Part model, mm, in its own coordinate system. A direction names the side the tool comes from. Give positions to 0.01 mm unless a question says otherwise; leave off trailing zeros. Loops run counter-clockwise (first coordinate to the right, second up) from the corner with the lowest first, then second, coordinate; pieces in that order, holes last. Notation, with made-up numbers: (20, 14.25) -> (28, 14.25) arc R8 ccw to (28, 24.25) -> close; hole circle Ø3 at (12, 44.5). An arc over 180 degrees is marked (long way). Write item = value, one per line.
from build123d import *

# Parameters (mm, degrees)
F1_R      = 47.625
F2_DEPTH  = 25.4
F0_R      = 88.9
F2_FACE_R = 47.625
F3_DEPTH  = 6.35
F4_R      = 5.08
F5_SIZE   = 2.54
F6_R      = 82.55
F6_R_2    = 57.15
F8_DEPTH  = 3.175
F7_R      = 41.275
F9_DEPTH  = 25.4
F10_R     = 1.524


with BuildPart() as f2:
    # F1 (on Top) → F2 (new body)
    with BuildSketch(Plane.XY):
        Circle(F1_R)
    extrude(amount=F2_DEPTH)

    # F0 (on Top) + F2_face (on face) → F3 (join)
    with BuildSketch(Plane.XY):
        Circle(F0_R)
    with BuildSketch(Plane.XY.offset(25.4)):
        Circle(F2_FACE_R)
    extrude(amount=-F3_DEPTH)

    # F4
    f4_edges = [f2.edges().sort_by_distance(p)[0] for p in [
        (-88.9, 0, -6.35),
    ]]
    fillet(f4_edges, radius=F4_R)

    # F5
    f5_edges = [f2.edges().sort_by_distance(p)[0] for p in [
        (-47.625, 0, 25.4),
    ]]
    chamfer(f5_edges, length=F5_SIZE)

    # F6 (on Top) → F8 (cut)
    with BuildSketch(Plane.XY):
        Circle(F6_R)
        Circle(F6_R_2, mode=Mode.SUBTRACT)
    extrude(amount=-F8_DEPTH, mode=Mode.SUBTRACT)

    # F7 (on Top) → F9 (cut)
    with BuildSketch(Plane.XY):
        Circle(F7_R)
    extrude(amount=F9_DEPTH, mode=Mode.SUBTRACT)

    # F10
    f10_edges = [f2.edges().sort_by_distance(p)[0] for p in [
        (-82.55, 0, -3.175),
        (-57.15, 0, -3.175),
        (-47.625, 0, 0),
    ]]
    fillet(f10_edges, radius=F10_R)


solid = f2.part
1) Drill centre lines: line 1 along Y through (x, z) = (0, -1); line 2 along Y through (x, z) = (0, 9) (3 decimals); line 3 along X through (y, z) = (-32.5, -1). Where is each one in solid material? Low to high. Write a range as [from, to].
Resolved:
line_1 = [-88.9, -82.55], [-57.15, 57.15], [82.55, 88.9]
line_2 = [-47.625, -41.275], [41.275, 47.625]
line_3 = [-82.75, -75.88], [-47.01, 47.01], [75.88, 82.75]
2) Pull direction X, two halves, no side cores. Call faces 3 (the face through (-1, 1, 0)), 4 (the face through (20, -37, 25.4)), 5 (the face through (-37.794, -28.979, 12.043)), 6 (the face through (-17.895, -80.587, -0.814)): pulls with the +X half, pulls with the -X half, needs draft (parallel to the pull), parting line crosses it, or undercut.
Resolved:
face_3 = undercut
face_4 = needs draft
face_5 = parting line crosses it
face_6 = undercut
3) Drop flat-ended pins along their axis: P1, Ø25, axis at x = -15.5, y = -20, coming from the +Z side; P2, Ø1.5, axis at x = 49.5, y = -51, coming from the +Z side (3 decimals). Give the stop position or say it passes through.
Resolved:
P1 = 0
P2 = -3.175
4) Slice it at C-C, the plane z = 10. List the corners of the cut face in (x, y) (3 decimals).
Resolved:
outline = circle Ø95.25 at (0, 0); hole circle Ø82.55 at (0, 0)
5) Which spindle directions (+Z, -Z, +X, -X, +Y, -Y) get a long thin tool onto all of the face, cutting with end or side? Do faces 1 (the face through (84.795, 26.703, -0.626)), 2 (the face through (54, 24, -3.175)). Say none if no direction does.
Resolved:
face_1 = +Z, -Z
face_2 = +Z
